from build123d import *

# Parameters (mm, degrees)
F1_DEPTH = 2
F2_R     = 0.99999
F3_R     = 0.99999


# Not quite as in the source:
# - a fillet or chamfer is up to 0.001 mm smaller than in the source, because OpenCascade refuses the exact size


with BuildPart() as f1:
    # F0 (on Front) → F1 (new body)
    with BuildSketch(Plane.XZ):
        Polygon((59.9, 0), (0, 0), (-59.9, 0), (-59.9, 35), (-61.9, 35), (-61.9, 0), (-79, 0), (-100, 0), (-102, 0), (-102, -80), (-99, -80), (-99, -12), (-89, -2), (-79, -2), (-79, -13), (-43, -13), (-43, -2), (-38.4, -2), (-38.4, -13), (-2.4, -13), (-2.4, -2), (0, -2), (2.4, -2), (2.4, -13), (38.4, -13), (38.4, -2), (43, -2), (43, -13), (79, -13), (79, -2), (91, -2), (91, 0), (79, 0), (61.9, 0), (61.9, 35), (59.9, 35), align=None)
    extrude(amount=F1_DEPTH)

    # F2 (radius 1 in the source; OpenCascade refuses exactly that, so slightly less here)
    f2_edges = [f1.edges().sort_by_distance(p)[0] for p in [
        (-84, -2, -2),
        (-84, 0, -2),
        (85, 0, -2),
        (85, -2, -2),
    ]]
    fillet(f2_edges, radius=F2_R)

    # F3 (radius 1 in the source; OpenCascade refuses exactly that, so slightly less here)
    f3_edges = [f1.edges().sort_by_distance(p)[0] for p in [
        (-40.7, -2, -2),
        (0, -2, -2),
        (40.7, -2, -2),
        (-40.7, 0, -2),
        (0, 0, -2),
        (40.7, 0, -2),
    ]]
    fillet(f3_edges, radius=F3_R)


solid = f1.part
Design review of the part built by this model. Coordinates are the model's own, in mm. Round coordinates to 2 decimals unless told otherwise and drop trailing zeros. Order: outer loops, then holes, each group sorted by start corner. A loop starts at its lowest first (then second) coordinate and runs counter-clockwise, first axis right, second up.
1) For L1, parallel to X at y = -1.8, z = -12.5; L2, parallel to X at y = -0.15, z = 14; L3, parallel to X at y = -1.8, z = -9, list the stretches that pass through material, from the lowest coordinate up.
The answers:
L1: x = -102 to -99, -79 to -43, -38.4 to -2.4, 2.4 to 38.4, 43 to 79
L2: x = -61.9 to -59.9, 59.9 to 61.9
L3: x = -102 to -96, -79 to -43, -38.4 to -2.4, 2.4 to 38.4, 43 to 79
2) Consider section B-B (z = -10). State the section outline as (x, y) points.
The answers:
outline: (-102, -2) - (-97, -2) - (-97, 0) - (-102, 0) - close; (-79, -2) - (-43, -2) - (-43, 0) - (-79, 0) - close; (-38.4, -2) - (-2.4, -2) - (-2.4, 0) - (-38.4, 0) - close; (2.4, -2) - (38.4, -2) - (38.4, 0) - (2.4, 0) - close; (43, -2) - (79, -2) - (79, 0) - (43, 0) - close
3) Draft analysis for pull direction X (two halves, no side actions). For faces 1 (the flat face through (-94, -1, -7)), 2 (the flat face through (-6, -2, -5)), state which applies: released by +X, released by -X, zero draft, split by the parting line, or undercut.
The answers:
face 1: undercut
face 2: zero draft
4) Clearance check with flat-ended pins moving along their axes: pin 1 Ø1 at (x, y) = (-0.5, -1) entering from -Z; pin 2 Ø0.6 at (y, z) = (-0.5, -9.5) entering from +X; pin 3 Ø12 at (x, z) = (-15, 8) entering from -Y; pin 4 Ø1 at (y, z) = (-1.5, 13.5) entering from +X. State where each tip first meets the part, or that it passes through.
The answers:
pin 1: stops at z = -2
pin 2: stops at x = 79
pin 3: passes through
pin 4: stops at x = 61.9
5) Consider section A-A (z = 15.5). State the section outline as (x, y) points.
The answers:
outline: (-61.9, -2) - (-59.9, -2) - (-59.9, 0) - (-61.9, 0) - close; (59.9, -2) - (61.9, -2) - (61.9, 0) - (59.9, 0) - close
